```python
from build123d import *

# Parameters (mm, degrees)
SKETCH1_R           = 15
BOSS_EXTRUDE1_DEPTH = 5
SKETCH2_W           = 23
SKETCH2_H           = 30
SKETCH2_W_2         = 23.001410072
BOSS_EXTRUDE2_DEPTH = 25
CUT_EXTRUDE1_REACH  = 168.903
SKETCH3_R           = 9.5


with BuildPart() as part:
    # Sketch1 → Boss-Extrude1 (new body)
    with BuildSketch(Plane.XY):
        with BuildLine():
            Line((-51.112042928, 5.109070396), (-28.112042928, 5.109070396))
            ThreePointArc((-28.112042928, 5.109070396), (35.387957072, -27.503737277), (98.887957072, 5.109070396))
            Line((98.887957072, 5.109070396), (121.887957072, 5.109070396))
            Line((121.887957072, 5.109070396), (121.887957072, -24.890929604))
            ThreePointArc((121.887957072, -24.890929604), (96.887957072, -49.890929604), (121.887957072, -74.890929604))
            Line((121.887957072, -74.890929604), (121.887957072, -104.890929604))
            Line((121.887957072, -104.890929604), (98.887957072, -104.890929604))
            ThreePointArc((98.887957072, -104.890929604), (35.387957072, -72.278121931), (-28.112042928, -104.890929604))
            Line((-28.112042928, -104.890929604), (-51.112042928, -104.890929604))
            Line((-51.112042928, -104.890929604), (-51.112042928, -74.890929604))
            ThreePointArc((-51.112042928, -74.890929604), (-26.112042928, -49.890929604), (-51.112042928, -24.890929604))
            Line((-51.112042928, -24.890929604), (-51.112042928, 5.109070396))
        make_face()
        with Locations((35.387957072, -49.890929604)):
            Circle(SKETCH1_R, mode=Mode.SUBTRACT)
        with Locations((72.887957072, -49.890929604)):
            Circle(SKETCH1_R, mode=Mode.SUBTRACT)
        with Locations((-2.112042928, -49.890929604)):
            Circle(SKETCH1_R, mode=Mode.SUBTRACT)
    extrude(amount=BOSS_EXTRUDE1_DEPTH)

    # Sketch2 → Boss-Extrude2 (add)
    with BuildSketch(Plane.XY.offset(5)):
        with Locations((-39.612042928, -9.890929604)):
            Rectangle(SKETCH2_W, SKETCH2_H)
        with Locations((110.387252036, -9.890929604)):
            Rectangle(SKETCH2_W_2, SKETCH2_H)
        with Locations((110.387252036, -89.890929604)):
            Rectangle(SKETCH2_W_2, SKETCH2_H)
        with Locations((-39.612042928, -89.890929604)):
            Rectangle(SKETCH2_W, SKETCH2_H)
    extrude(amount=BOSS_EXTRUDE2_DEPTH)

    # Cut-Extrude1: up to this face of the body (flat: up to its plane)
    cut_extrude1_end = Plane(part.part.faces().sort_by_distance((-39.612042928, 5.109070396, 15))[0])
    # Sketch3 → Cut-Extrude1 (cut, up to the picked face)
    with BuildSketch(Plane.XZ.offset(104.890929604), mode=Mode.PRIVATE) as cut_extrude1_sk1:
        with Locations(Location((110.387604554, 15, 0), (0, 0, 270))):
            Circle(SKETCH3_R)
    cut_extrude1_tool1 = split(extrude(cut_extrude1_sk1.sketch, amount=-CUT_EXTRUDE1_REACH, mode=Mode.PRIVATE), bisect_by=cut_extrude1_end, keep=Keep.BOTH, mode=Mode.PRIVATE)
    # Sketch3 → Cut-Extrude1 (cut, up to the picked face)
    with BuildSketch(Plane.XZ.offset(104.890929604), mode=Mode.PRIVATE) as cut_extrude1_sk2:
        with Locations(Location((-39.612042928, 15, 0), (0, 0, 270))):
            Circle(SKETCH3_R)
    cut_extrude1_tool2 = split(extrude(cut_extrude1_sk2.sketch, amount=-CUT_EXTRUDE1_REACH, mode=Mode.PRIVATE), bisect_by=cut_extrude1_end, keep=Keep.BOTH, mode=Mode.PRIVATE)
    add(cut_extrude1_tool1.solids().sort_by(Axis((110.387605, -104.89093, 15), (0, 1, 0)))[0], mode=Mode.SUBTRACT)
    add(cut_extrude1_tool2.solids().sort_by(Axis((-39.612043, -104.89093, 15), (0, 1, 0)))[0], mode=Mode.SUBTRACT)


solid = part.part
```
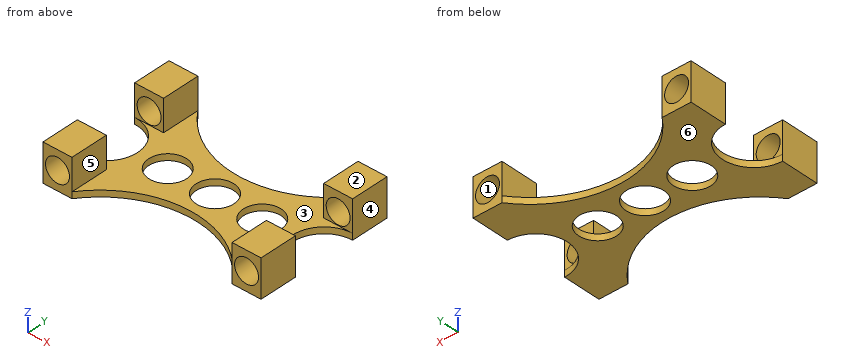
Verification items for the finished model (mm, model axes). Face numbers are marked on the shaded views. A direction names the side the tool comes from. Coordinates: 2 decimals unless noted, no trailing zeros. Loops run counter-clockwise (first coordinate to the right, second up) from the corner with the lowest first, then second, coordinate; pieces in that order, holes last. Notation, with made-up numbers: (77.25, 20) -> (91.25, 20) arc R20 ccw to (91.25, 59) -> close; hole circle Ø3 at (0, -18). An arc over 180 degrees is marked (long way). Answer in a Markdown table with one row per item. Add a question column.
1. Section check A-A, the plane z = 15. Give the number of separate pieces and of enclosed holes in the cut face, then the cut area to 3 significant figures.
2. Material ranges on probe 1 along X at (y, z) = (-13.25, 15); probe 2 along X at (y, z) = (-79, 21.75); probe 3 along X at (y, z) = (-76, 28.75), recorded low to high. Write a range as [from, to].
3. Section check D-D, the plane x = 46. Enter the section's corners in (y, z), then the cut area to 3 significant figures.
4. Draft check along X on the marked faces 1, 2, 3 and 4. Enter one of: +X half, -X half, draft (parallel to the pull), parting line (faces both ways), or undercut.
5. Section check C-C, the plane y = -22. Enter the section's corners in (x, z), then the cut area to 3 significant figures.
6. Access from +Z, -Z, +X, -X, +Y, -Y to the whole of each face (thin tool, end or side, straight path). Record for the marked faces 5 and 6.
7. Section check B-B, the plane x = 81.5. Enter the section's corners in (y, z), then the cut area to 3 significant figures.
8. Depth check by flat-ended pin: P1, Ø8, axis at x = 86.5, y = -81, coming from the +Z side. Enter the tip coordinate at first touch or a pass-through.
Derived:
| question | item | result |
|---|---|---|
| 1 | separate pieces | 8 |
| 1 | enclosed holes | 0 |
| 1 | area | 480 mm² |
| 2 | probe 1 | x = [-51.11, -49.11], [-30.11, -28.11], [98.89, 100.89], [119.89, 121.89] |
| 2 | probe 2 | x = [-51.11, -46.3], [-32.93, -28.11], [98.89, 103.7], [117.07, 121.89] |
| 2 | probe 3 | x = [-51.11, -28.11], [98.89, 121.89] |
| 3 | outline | (-73, 0) -> (-60.49, 0) -> (-60.49, 5) -> (-73, 5) -> close; (-39.29, 0) -> (-26.78, 0) -> (-26.78, 5) -> (-39.29, 5) -> close |
| 3 | area | 125 mm² |
| 4 | face 1 | undercut |
| 4 | face 2 | draft |
| 4 | face 3 | undercut |
| 4 | face 4 | +X half |
| 5 | outline | (-51.11, 0) -> (6.58, 0) -> (6.58, 5) -> (-28.11, 5) -> (-28.11, 30) -> (-51.11, 30) -> close; (64.19, 0) -> (121.89, 0) -> (121.89, 30) -> (98.89, 30) -> (98.89, 5) -> (64.19, 5) -> close; hole circle Ø19 at (-39.61, 15); hole circle Ø19 at (110.39, 15) |
| 5 | area | 1,160 mm² |
| 6 | face 5 | +Z, +Y, -Y |
| 6 | face 6 | -Z, +X, -X, +Y, -Y |
| 7 | outline | (-87.34, 0) -> (-62.17, 0) -> (-62.17, 5) -> (-87.34, 5) -> close; (-37.61, 0) -> (-12.44, 0) -> (-12.44, 5) -> (-37.61, 5) -> close |
| 7 | area | 252 mm² |
| 8 | P1 | stops at z = 5 |
